from build123d import *


with BuildPart() as part:
    # Sketch1 → Revolve1 (revolve)
    with BuildSketch(Plane(origin=(0, 0, 0), x_dir=(0, 0, -1), z_dir=(1, 0, 0)), mode=Mode.PRIVATE) as revolve1_sk:
        with BuildLine():
            Line((-22.5, 50), (22.5, 50))
            Line((22.5, 50), (22.5, 47.5))
            Line((22.5, 47.5), (9.264260449, 43.5))
            ThreePointArc((9.264260449, 43.5), (6.182612881, 41.333250628), (5, 37.756550844))
            Line((5, 37.756550844), (5, 28.202513909))
            ThreePointArc((5, 28.202513909), (6.142274104, 24.680795703), (9.134166373, 22.5))
            Line((9.134166373, 22.5), (29, 16))
            Line((29, 16), (29, 12.5))
            Line((29, 12.5), (-29, 12.5))
            Line((-29, 12.5), (-29, 16))
            Line((-29, 16), (-9.134166373, 22.5))
            ThreePointArc((-9.134166373, 22.5), (-6.142274104, 24.680795703), (-5, 28.202513909))
            Line((-5, 28.202513909), (-5, 37.756550844))
            ThreePointArc((-5, 37.756550844), (-6.182612881, 41.333250628), (-9.264260449, 43.5))
            Line((-9.264260449, 43.5), (-22.5, 47.5))
            Line((-22.5, 47.5), (-22.5, 50))
        make_face()
    revolve(revolve1_sk.sketch.rotate(Axis((0, 0, 41.444357118), (0, 0, -1)), 90), axis=Axis((0, 0, 41.444357118), (0, 0, -1)))


solid = part.part
Part model, mm, in its own coordinate system. A direction names the side the tool comes from. Give positions to 0.01 mm unless a question says otherwise; leave off trailing zeros. Write each loop counter-clockwise with the first axis right and the second up, starting at its lowest first coordinate (ties: lowest second). Pieces come first, ordered by that corner, then holes.
1) Cut at D-D on z = 21. Write the cut outline in (x, y).
Resolved:
outline: circle Ø100 at (0, 0); circle Ø37.24 at (0, 0); hole circle Ø94.09 at (0, 0); hole circle Ø25 at (0, 0)
2) Two-plate mould, pull along Y, no slides. Class faces 1 (the face through (14, 25, 5)), 2 (the face through (-14, 25, -5)), 3 (the face through (47.69, -15.02, -0.32)), 4 (the face through (-44.2, 18.3, 22.5)): released by +Y, released by -Y, zero draft, split by the parting line, or undercut.
Resolved:
face 1: undercut
face 2: undercut
face 3: split by the parting line
face 4: zero draft
3) Probe L1, parallel to Y at x = 0, z = -9; L2, parallel to Y at x = 0, z = 4; L3, parallel to Y at x = 0, z = 16.5. List the from-to ranges inside material, lowest first.
Resolved:
L1: y = -50 to -43.41, -22.55 to -12.5, 12.5 to 22.55, 43.41 to 50
L2: y = -50 to -12.5, 12.5 to 50
L3: y = -50 to -45.69, -20.09 to -12.5, 12.5 to 20.09, 45.69 to 50
4) Pin check, flat tips, straight feed: pin 1 (10 mm diameter, centred on x = -25.5, y = -22.5, fed in from -Z); pin 2 (3 mm diameter, centred on y = -17.5, z = 7, fed in from +X); pin 3 (2 mm diameter, centred on y = -25.5, z = -9, fed in from +X); pin 4 (22.5 mm diameter, centred on x = 0, y = 0, fed in from -Z). Stop position of each tip, or through.
Resolved:
pin 1: stops at z = -5.13
pin 2: stops at x = 47.37
pin 3: stops at x = 43.59
pin 4: passes through
5) Cut at C-C on z = -16. Write the cut outline in (x, y).
Resolved:
outline: circle Ø100 at (0, 0); circle Ø40.51 at (0, 0); hole circle Ø91.07 at (0, 0); hole circle Ø25 at (0, 0)
6) Which spindle directions (+Z, -Z, +X, -X, +Y, -Y) get a long thin tool onto all of the face, cutting with end or side? Do faces 5 (the face through (-10, 8, -29)), 6 (the face through (44.2, 18.3, -22.5)). Say none if no direction does.
Resolved:
face 5: -Z, +X, -X, +Y, -Y
face 6: -Z
